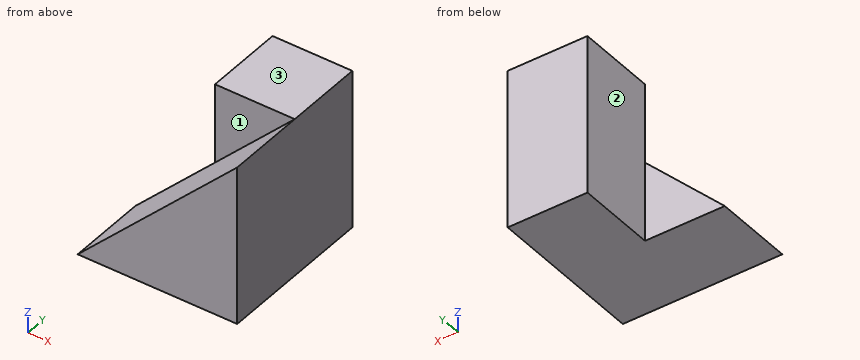
```python
from build123d import *

# Parameters (mm, degrees)
SKETCH1_W           = 40
SKETCH1_H           = 20
BOSS_EXTRUDE1_DEPTH = 40
SKETCH2_W           = 20
SKETCH2_H           = 20
BOSS_EXTRUDE2_DEPTH = 40
CUT_EXTRUDE1_DEPTH  = 20
SKETCH4_W           = 40
SKETCH4_H           = 20
CUT_EXTRUDE2_DEPTH  = 35
CUT_EXTRUDE3_DEPTH  = 35
SKETCH6_W           = 20
SKETCH6_H           = 40
BOSS_EXTRUDE3_DEPTH = 20


with BuildPart() as part:
    # Sketch1 → Boss-Extrude1 (new body)
    with BuildSketch(Plane.XY):
        with Locations((20, 10)):
            Rectangle(SKETCH1_W, SKETCH1_H)
    extrude(amount=BOSS_EXTRUDE1_DEPTH)

    # Sketch2 → Boss-Extrude2 (add)
    with BuildSketch(Plane.XY.offset(40)):
        with Locations((30, 30)):
            Rectangle(SKETCH2_W, SKETCH2_H)
    extrude(amount=-BOSS_EXTRUDE2_DEPTH)

    # Sketch3 → Cut-Extrude1 (cut)
    with BuildSketch(Plane(origin=(0, 40, 0), x_dir=(1, 0, 0), z_dir=(0, 1, 0))):
        Polygon((20, -40), (40, -20), (40, -40), align=None)
    extrude(amount=-CUT_EXTRUDE1_DEPTH, mode=Mode.SUBTRACT)

    # Sketch4 → Cut-Extrude2 (cut)
    with BuildSketch(Plane.ZY.offset(-20)):
        with Locations((20, 30)):
            Rectangle(SKETCH4_W, SKETCH4_H)
    extrude(amount=-CUT_EXTRUDE2_DEPTH, mode=Mode.SUBTRACT)

    # Sketch5 → Cut-Extrude3 (cut)
    with BuildSketch(Plane(origin=(0, 20, 0), x_dir=(1, 0, 0), z_dir=(0, 1, 0))):
        Polygon((0, 0), (40, -40), (0, -40), align=None)
    extrude(amount=-CUT_EXTRUDE3_DEPTH, mode=Mode.SUBTRACT)

    # Sketch6 → Boss-Extrude3 (add)
    with BuildSketch(Plane(origin=(0, 20, 0), x_dir=(1, 0, 0), z_dir=(0, 1, 0))):
        with Locations((30, -20)):
            Rectangle(SKETCH6_W, SKETCH6_H)
    extrude(amount=BOSS_EXTRUDE3_DEPTH)


solid = part.part
```
For this review, take the finished solid that the model builds, in its own axes (mm). Face numbers are marked on the shaded views. A direction names the side the tool comes from. Round coordinates to 2 decimals unless told otherwise and drop trailing zeros. Order: outer loops, then holes, each group sorted by start corner. A loop starts at its lowest first (then second) coordinate and runs counter-clockwise, first axis right, second up.
Q1. Machinability: for the marked faces 1, 2 and 3, which of the approach directions +Z, -Z, +X, -X, +Y, -Y give a long, thin tool a straight path to every point of the face, cutting with its end or side? Answer none if there is none.
Findings below:
face 1: +Z, -X, -Y
face 2: +Z, -Z, -X, +Y
face 3: +Z, +X, -X, +Y, -Y
Q2. We need section B-B, the plane z = 10. Give the boundary of the cut face in (x, y).
Findings below:
outline: (10, 0) - (40, 0) - (40, 40) - (20, 40) - (20, 20) - (10, 20) - close
Q3. We need section C-C, the plane y = 4.5. Give the boundary of the cut face in (x, z).
Findings below:
outline: (0, 0) - (40, 0) - (40, 40) - close
Q4. Insertion check: P1, Ø22, axis at x = 7.5, z = 7.5, coming from the +Y side; P2, Ø1.5, axis at y = 16, z = 7, coming from the -X side; P3, Ø10, axis at y = 25.5, z = 11, coming from the -X side. Each pin has a flat end and moves straight along its axis. Give the tip position at first contact, or say it passes through.
Findings below:
P1: stops at y = 20
P2: stops at x = 6.25
P3: stops at x = 20
Q5. Wall thickness on line 1 (X direction, y = 33, z = 34.5); line 2 (Z direction, x = 22.5, y = 2.5): over which ranges is each line inside the solid? List them lowest first.
Findings below:
line 1: x = 20 to 40
line 2: z = 0 to 22.5
Q6. We need section D-D, the plane x = 10.5. Give the boundary of the cut face in (y, z), plus the area to 3 significant figures.
Findings below:
outline: (0, 0) - (20, 0) - (20, 10.5) - (0, 10.5) - close
area: 210 mm2
Q7. We need section A-A, the plane x = 25. Give the boundary of the cut face in (y, z).
Findings below:
outline: (0, 0) - (40, 0) - (40, 40) - (20, 40) - (20, 25) - (0, 25) - close
